```python
from build123d import *

# Parameters (mm, degrees)
SKETCH1_W                    = 54.61
SKETCH1_H                    = 54.61
BOSS_EXTRUDE1_DEPTH          = 6.35
F_10_0_1935_DIAMETER_HOLE1_D = 4.9149
SKETCH7_R                    = 27.305
BOSS_EXTRUDE2_DEPTH          = 69.85
SKETCH8_R                    = 3.175
BOSS_EXTRUDE3_DEPTH          = 19.05
BOSS_EXTRUDE4_START          = 19.05
SKETCH9_R                    = 3.175
BOSS_EXTRUDE4_DEPTH          = 19.05


with BuildPart() as part:
    # Sketch1 → Boss-Extrude1 (new body)
    with BuildSketch(Plane.XY):
        Rectangle(SKETCH1_W, SKETCH1_H)
    extrude(amount=BOSS_EXTRUDE1_DEPTH)

    # #10 (0.1935) Diameter Hole1 (through all)
    with Locations(Plane.XY.offset(6.35)):
        with Locations((-23.5458, 23.5458), (23.510742074, 23.5458), (23.510742074, -23.510742074), (-23.5458, -23.510742074)):
            Hole(F_10_0_1935_DIAMETER_HOLE1_D / 2)

    # Sketch7 → Boss-Extrude2 (add)
    with BuildSketch(Plane(origin=(0, 0, 0), x_dir=(-1, 0, 0), z_dir=(0, 0, -1))):
        Circle(SKETCH7_R)
    extrude(amount=BOSS_EXTRUDE2_DEPTH)

    # Sketch8 → Boss-Extrude3 (add)
    with BuildSketch(Plane(origin=(0, 0, -69.85), x_dir=(-1, 0, 0), z_dir=(0, 0, -1))):
        with Locations(Location((0, 0, 0), (0, 0, 180))):
            Circle(SKETCH8_R)
    extrude(amount=BOSS_EXTRUDE3_DEPTH)

    # Sketch9 → Boss-Extrude4 (add)
    with BuildSketch(Plane.XY.offset(6.35).offset(BOSS_EXTRUDE4_START)):
        Circle(SKETCH9_R)
    extrude(amount=-BOSS_EXTRUDE4_DEPTH)


solid = part.part
```
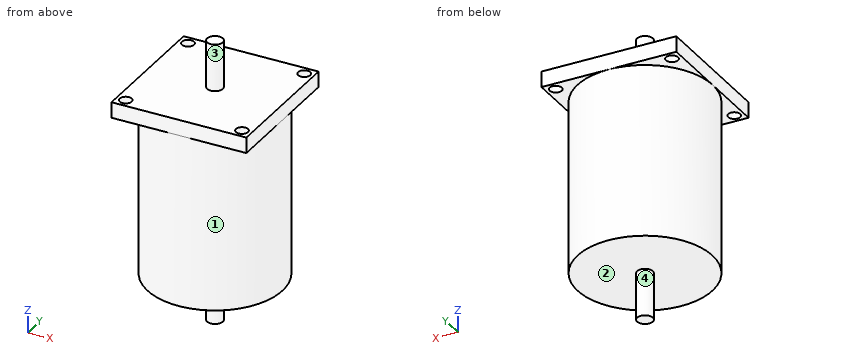
The listing builds one solid part. Answer for the finished solid, in the listing's coordinates (mm). Face numbers are marked on the shaded views. A direction names the side the tool comes from. Give positions to 0.01 mm unless a question says otherwise; leave off trailing zeros. Order: outer loops, then holes, each group sorted by start corner. A loop starts at its lowest first (then second) coordinate and runs counter-clockwise, first axis right, second up. Notation, with made-up numbers: M 52,59 L 91,59 A5 cw 91,68 Z; hole C -19.5,23 d3. An arc over 180 degrees is marked long. Put each result on its own line as item: value. Start each with the question number.
Item 1: Which of the six approach directions +Z, -Z, +X, -X, +Y, -Y give full straight-line access (tool end or side, diameter ignored) to the marked faces 3 and 4?
Item 2: Find the intervals of material crossed by line 1 along X through (y, z) = (1, -21); line 2 along Z through (x, y) = (-1.5, -9.5); line 3 along Y through (x, z) = (21, -57), in increasing order.
Item 3: Flat-ended cylindrical pins translate along their axes: P1, Ø3, axis at x = 20.5, z = -63.5, coming from the -Y side; P2, Ø3, axis at x = 19, z = -47, coming from the -Y side; P3, Ø5, axis at x = -10, y = 15.5, coming from the +Z side. Find the tip coordinate at first contact, or state that the pin passes through.
Item 4: The part is cut by section B-B, the plane y = -2. Determine the outline of the cut face in (x, z) (3 decimals).
Item 5: For a pull along Y with two mould halves and no side action, classify the marked faces 1 and 2 as +Y half, -Y half, draft (parallel to the pull), parting line (faces both ways), or undercut.
Item 6: The part is cut by section D-D, the plane y = 12. Determine the outline of the cut face in (x, z) (3 decimals).
Item 7: The part is cut by section A-A, the plane x = 16. Determine the outline of the cut face in (y, z) (3 decimals), and give its area (3 significant figures).
Item 8: The part is cut by section C-C, the plane z = -29.5. Determine the outline of the cut face in (x, y) (3 decimals).
Answer key:
1. face 3: +Z
1. face 4: -Z
2. line 1: x = -27.29 to 27.29
2. line 2: z = -69.85 to 6.35
2. line 3: y = -17.45 to 17.45
3. P1: stops at y = -19.61
3. P2: stops at y = -20.96
3. P3: stops at z = 6.35
4. outline: M -27.305,0 L -27.232,0 L -27.232,-69.85 L -2.466,-69.85 L -2.466,-88.9 L 2.466,-88.9 L 2.466,-69.85 L 27.232,-69.85 L 27.232,0 L 27.305,0 L 27.305,6.35 L 2.466,6.35 L 2.466,25.4 L -2.466,25.4 L -2.466,6.35 L -27.305,6.35 Z
5. face 1: parting line
5. face 2: draft
6. outline: M -27.305,0 L -24.527,0 L -24.527,-69.85 L 24.527,-69.85 L 24.527,0 L 27.305,0 L 27.305,6.35 L -27.305,6.35 Z
7. outline: M -27.305,0 L -22.126,0 L -22.126,-69.85 L 22.126,-69.85 L 22.126,0 L 27.305,0 L 27.305,6.35 L -27.305,6.35 Z
7. area: 3,440 mm²
8. outline: C 0,0 d54.61
